Build history of the part. All positions in model axes, mm. A direction names the side the tool comes from. Round coordinates to 2 decimals unless told otherwise and drop trailing zeros. Write each loop counter-clockwise with the first axis right and the second up, starting at its lowest first coordinate (ties: lowest second). Pieces come first, ordered by that corner, then holes. Notation, with made-up numbers: (19, -25.75) -> (45, -25.75) arc R11 ccw to (45, -14.75) -> close; hole circle Ø7 at (-34, 42). An arc over 180 degrees is marked (long way). Answer in a Markdown table with one row per item.
```python
from build123d import *

# Parameters (mm, degrees)
BOSS_EXTRUDE1_DEPTH = 7
CUT_EXTRUDE1_DEPTH  = 8
SKETCH5_W           = 15
SKETCH5_H           = 3
CUT_EXTRUDE3_DEPTH  = 10
SKETCH6_W           = 12.1
SKETCH6_H           = 5.1
CUT_EXTRUDE4_DEPTH  = 2.1


with BuildPart() as part:
    # Sketch1 → Boss-Extrude1 (new body)
    with BuildSketch(Plane(origin=(0, 0, 0), x_dir=(1, 0, 0), z_dir=(0, 1, 0))):
        with BuildLine():
            Line((7, 21.2), (-21.2, 21.2))
            ThreePointArc((-21.2, 21.2), (-6.209336239, 14.990663761), (0, 0))
            Line((0, 0), (7, 0))
            Line((7, 0), (7, 21.2))
        make_face()
    extrude(amount=BOSS_EXTRUDE1_DEPTH)

    # Sketch2 → Cut-Extrude1 (cut, through all)
    with BuildSketch(Plane(origin=(0, 7, 0), x_dir=(1, 0, 0), z_dir=(0, 1, 0))):
        with BuildLine():
            Line((-9.2, 17.47684182), (-9.2, 21.2))
            Line((-9.2, 21.2), (-21.2, 21.2))
            ThreePointArc((-21.2, 21.2), (-14.917844581, 20.247827619), (-9.2, 17.47684182))
        make_face()
    extrude(amount=-CUT_EXTRUDE1_DEPTH, mode=Mode.SUBTRACT)

    # Sketch5 → Cut-Extrude3 (cut)
    with BuildSketch(Plane(origin=(0, 0, 0), x_dir=(0, 0, -1), z_dir=(1, 0, 0))):
        with Locations((9.5, 4.5)):
            Rectangle(SKETCH5_W, SKETCH5_H)
    extrude(amount=-CUT_EXTRUDE3_DEPTH, mode=Mode.SUBTRACT)

    # Sketch6 → Cut-Extrude4 (cut)
    with BuildSketch(Plane(origin=(7, 0, 0), x_dir=(0, 0, -1), z_dir=(1, 0, 0))):
        with Locations((7.05, 3.55)):
            Rectangle(SKETCH6_W, SKETCH6_H)
    extrude(amount=-CUT_EXTRUDE4_DEPTH, mode=Mode.SUBTRACT)


with BuildPart() as body_2:
    # Mirror1: mirrored copy
    add(part.part.mirror(Plane(origin=(0, 7, 0), x_dir=(1, 0, 0), z_dir=(0, 0, -1))))


solid = body_2.part
```
Q1. Saw through at B-B on y = 5.25. Write the cut outline in (x, z).
A:
| item | result |
|---|---|
| outline | (-9.2, 17.48) arc R21.2 cw to (-8.53, 17) -> (0, 17) -> (0, 2) -> (-0.09, 2) arc R21.2 cw to (0, 0) -> (7, 0) -> (7, 1) -> (4.9, 1) -> (4.9, 13.1) -> (7, 13.1) -> (7, 21.2) -> (-9.2, 21.2) -> close |
Q2. Which spindle directions (+Z, -Z, +X, -X, +Y, -Y) get a long thin tool onto all of the face, cutting with end or side? Do faces 4 (the flat face through (3, 3, 0)), 5 (the flat face through (6, 6.1, 7)). Say none if no direction does.
A:
| item | result |
|---|---|
| face 4 | -Z, +X, -X, +Y, -Y |
| face 5 | +X |
Q3. Saw through at D-D on x = -5.75. Write the cut outline in (y, z), plus the area to 3 significant figures.
A:
| item | result |
|---|---|
| outline | (0, 14.52) -> (3, 14.52) -> (3, 17) -> (6, 17) -> (6, 14.52) -> (7, 14.52) -> (7, 21.2) -> (0, 21.2) -> close |
| area | 39.3 mm² |
Q4. Saw through at A-A on x = 5.5. Write the cut outline in (y, z).
A:
| item | result |
|---|---|
| outline | (0, 0) -> (7, 0) -> (7, 21.2) -> (0, 21.2) -> close; hole (1, 1) -> (6.1, 1) -> (6.1, 13.1) -> (1, 13.1) -> close |
Q5. Wall check: line 1 (Y direction, x = -3, z = 11); line 2 (Z direction, x = 5.75, y = 3.5); line 3 (X direction, y = 5, z = 14.5). Give the ranges that are in metal, low to high. Write a range as [from, to].
A:
| item | result |
|---|---|
| line 1 | [0, 3], [6, 7] |
| line 2 | [0, 1], [13.1, 21.2] |
| line 3 | [0, 7] |
Q6. Two-plate mould, pull along Z, no slides. Class faces 1 (the flat face through (-9.2, 4, 19)), 2 (the flat face through (0, 5, 9)), 3 (the cylindrical face through (-2.508, 2.673, 10.002)): released by +Z, released by -Z, zero draft, split by the parting line, or undercut.
A:
| item | result |
|---|---|
| face 1 | zero draft |
| face 2 | undercut |
| face 3 | released by -Z |
Q7. Drop flat-ended pins along their axis: P1, Ø2, axis at y = 5.5, z = 5.5, coming from the -X side; P2, Ø1.5, axis at y = 4.5, z = 12.5, coming from the -X side; P3, Ø0.9, axis at x = -6.5, y = 5, coming from the -Z side. Give the stop position or say it passes through.
A:
| item | result |
|---|---|
| P1 | x = -0.98 |
| P2 | x = 0 |
| P3 | z = 17 |
Q8. Saw through at C-C on z = 2.25. Write the cut outline in (x, y), plus the area to 3 significant figures.
A:
| item | result |
|---|---|
| outline | (-0.12, 0) -> (7, 0) -> (7, 1) -> (4.9, 1) -> (4.9, 6.1) -> (7, 6.1) -> (7, 7) -> (-0.12, 7) -> (-0.12, 6) -> (0, 6) -> (0, 3) -> (-0.12, 3) -> close |
| area | 38.8 mm² |
